Print and shaded views of the part. All mm, measured from the part's lowest x, y and z. A direction names the side the tool comes from. Round coordinates to 2 decimals unless told otherwise and drop trailing zeros. Order: outer loops, then holes, each group sorted by start corner. A loop starts at its lowest first (then second) coordinate and runs counter-clockwise, first axis right, second up.
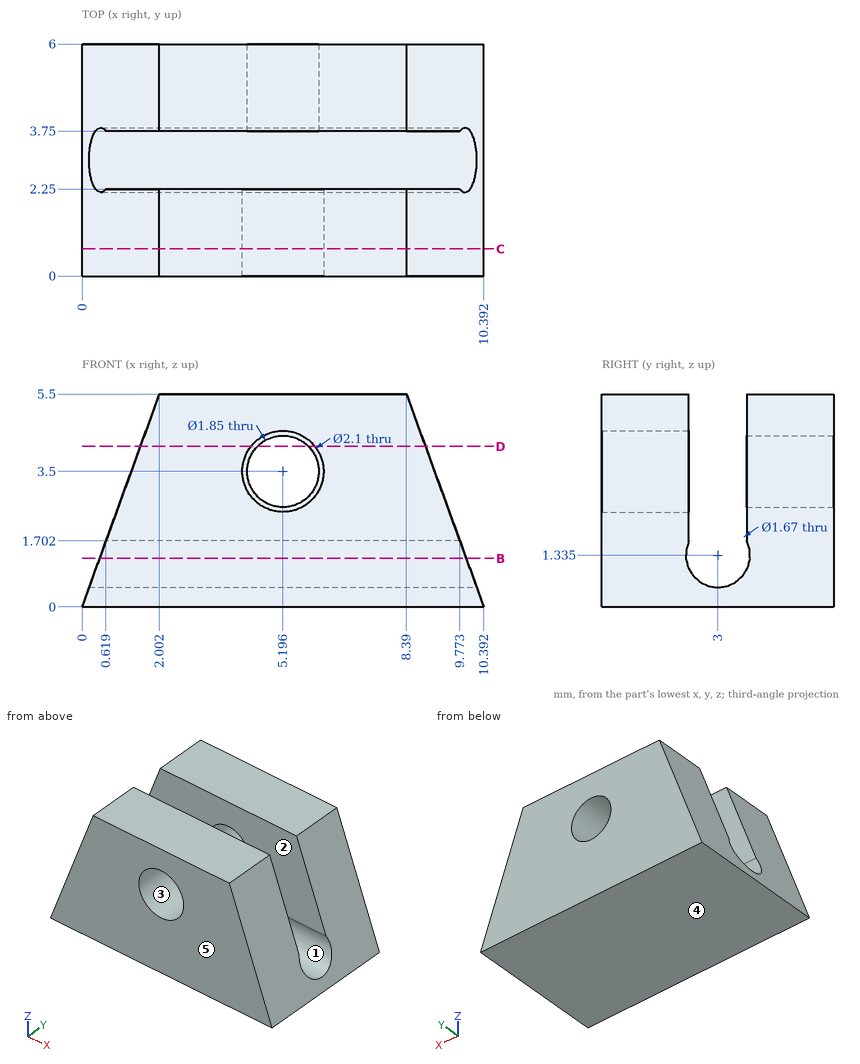
1. Drill centre lines: line 1 (Y direction, x = 5.5, z = 4.65); line 2 (Z direction, x = 6.5, y = 3); line 3 (X direction, y = 0.85, z = 3.5) (1 decimal). Where is each one in solid material? Low to high.
2. Cut at D-D, the plane z = 4.15. Give the number of separate pieces and of enclosed holes in the cut face, and give its area (3 significant figures).
3. Tool access for the marked faces 1 and 2: list every direction of +Z, -Z, +X, -X, +Y, -Y with a clear straight run to the whole face (end or side of a thin tool).
4. Cut at C-C, the plane y = 0.7. Write the cut outline in (x, z).
5. Pin check, flat tip, straight feed: P1, Ø1.5, axis at y = 1, z = 2, coming from the -X side (1 decimal). Stop position of the tip, or through.
6. Cut at B-B, the plane z = 1.25. Write the cut outline in (x, y) (1 decimal).
7. Mould opens along Z. For the marked faces 3, 4 and 5 say: released by +Z, released by -Z, zero draft, split by the parting line, or undercut.
Outcome:
1. line 1: y = 0 to 2.25, 3.75 to 6
1. line 2: z = 0 to 0.5
1. line 3: x = 1.3 to 4.1, 6.2 to 9.1
2. separate pieces: 4
2. enclosed holes: 0
2. area: 26.5 mm2
3. face 1: +X, -X
3. face 2: +Z, +X, -X
4. outline: (0, 0) - (10.39, 0) - (8.39, 5.5) - (2, 5.5) - close; hole circle Ø2.1 at (5.2, 3.5)
5. P1: stops at x = 0.5
6. outline: (0.5, 0) - (9.9, 0) - (9.9, 2.2) - (0.5, 2.2) - close; (0.5, 3.8) - (9.9, 3.8) - (9.9, 6) - (0.5, 6) - close
7. face 3: undercut
7. face 4: released by -Z
7. face 5: zero draft
